from build123d import *

# Parameters (mm, degrees)
SKETCH1_R               = 15
SKETCH1_R_2             = 5
EXTRUDE_THIN1_DEPTH     = 50
SKETCH2_W               = 70
SKETCH2_H               = 30
BOSS_EXTRUDE1_DEPTH     = 16
SKETCH3_R               = 6
BOSS_EXTRUDE2_DEPTH     = 10
EXTRUDE_THIN2_DEPTH     = 12.5
FILLET1_R               = 30
BOSS_EXTRUDE3_DEPTH     = 10
CUT_EXTRUDE1_DEPTH      = 172.116081143
CUT_EXTRUDE1_DEPTH_BACK = 172.116081143
SKETCH6_R               = 10


with BuildPart() as part:
    # Sketch1 → Extrude-Thin1 (new, symmetric)
    with BuildSketch(Plane(origin=(0, 0, 0), x_dir=(0, 0, -1), z_dir=(1, 0, 0))):
        Circle(SKETCH1_R)
        Circle(SKETCH1_R_2, mode=Mode.SUBTRACT)
    extrude(amount=EXTRUDE_THIN1_DEPTH, both=True)

    # Sketch2 → Boss-Extrude1 (add)
    with BuildSketch(Plane(origin=(0, 0, 0), x_dir=(1, 0, 0), z_dir=(0, 1, 0))):
        Rectangle(SKETCH2_W, SKETCH2_H)
    extrude(amount=BOSS_EXTRUDE1_DEPTH)

    # Sketch3 → Boss-Extrude2 (add)
    with BuildSketch(Plane(origin=(0, 16, 0), x_dir=(1, 0, 0), z_dir=(0, 1, 0))):
        with Locations(Location((0, 0, 0), (0, 0, 270))):
            Circle(SKETCH3_R)
    extrude(amount=BOSS_EXTRUDE2_DEPTH)

    # Sketch4 → Extrude-Thin2 (add, symmetric)
    with BuildSketch(Plane(origin=(0, 0, 0), x_dir=(0, 0, -1), z_dir=(1, 0, 0))):
        Polygon((-14.175668382, 24.036944014), (10.301514998, 24.036944014), (42.733043078, 53.23603901), (154.74701088, 53.23603901), (154.74701088, 50.23603901), (43.884565313, 50.23603901), (11.453037232, 21.036944014), (-14.175668382, 21.036944014), align=None)
    extrude(amount=EXTRUDE_THIN2_DEPTH, both=True)

    # Fillet1
    # the kernel refuses this fillet: 30 mm, written as the material it adds along each edge
    with BuildSketch(Plane(origin=(12.5, 50.23603901, -43.884565313), x_dir=(0, -0.6691004351822665, 0.7431719906178524), z_dir=(-1, 0, 0))) as fillet1_piece_1:
        with BuildLine():
            CenterArc((FILLET1_R * 0.383840744794, -FILLET1_R), FILLET1_R, 90, 41.997673873)
            Line((-FILLET1_R * 0.285259690389, -FILLET1_R * 0.256828009382), (0, 0))
            Line((0, 0), (FILLET1_R * 0.383840744794, 0))
        make_face()
    extrude(amount=25)
    with BuildSketch(Plane(origin=(12.5, 24.036944014, -10.301514998), x_dir=(0, 0, 1), z_dir=(-1, 0, 0))) as fillet1_piece_2:
        with BuildLine():
            CenterArc((FILLET1_R * 0.383840744794, FILLET1_R), FILLET1_R, 228.002326127, 41.997673873)
            Line((-FILLET1_R * 0.285259690389, FILLET1_R * 0.256828009382), (0, 0))
            Line((0, 0), (FILLET1_R * 0.383840744794, 0))
        make_face()
    extrude(amount=25)
    # the kernel refuses this fillet: 30 mm, written as the material it takes off along each edge
    with BuildSketch(Plane(origin=(41.28805586, 53.23603901, -42.733043078), x_dir=(0, -0.6691004351822663, 0.7431719906178528), z_dir=(-1, 0, 0))) as fillet1_2_piece_1:
        with BuildLine():
            CenterArc((FILLET1_R * 0.383840744794, -FILLET1_R), FILLET1_R, 90, 41.997673873)
            Line((-FILLET1_R * 0.285259690389, -FILLET1_R * 0.256828009382), (0, 0))
            Line((0, 0), (FILLET1_R * 0.383840744794, 0))
        make_face()
    extrude(amount=82.576111719, mode=Mode.SUBTRACT)
    with BuildSketch(Plane(origin=(-41.28805586, 21.036944014, -11.453037232), x_dir=(0, 0, 1), z_dir=(1, 0, 0))) as fillet1_2_piece_2_section:
        with BuildLine():
            CenterArc((FILLET1_R * 0.383840744794, -FILLET1_R), FILLET1_R, 90, 41.997673873)
            Line((-FILLET1_R * 0.285259690389, -FILLET1_R * 0.256828009382), (0, 0))
            Line((0, 0), (FILLET1_R * 0.383840744794, 0))
        make_face()
    fillet1_2_piece_2 = extrude(amount=82.576111719, mode=Mode.PRIVATE)
    fillet1_2_piece_2 = fillet1_2_piece_2 - Plane(origin=(0, 22.678661346, 0), x_dir=(0, 0, 1), z_dir=(0, -1, 0)) * Cylinder(6, 212, mode=Mode.PRIVATE)
    add(fillet1_2_piece_2, mode=Mode.SUBTRACT)

    # Sketch5 → Boss-Extrude3 (add)
    with BuildSketch(Plane(origin=(50, 0, 0), x_dir=(0, 0, -1), z_dir=(1, 0, 0))):
        Polygon((-20.207259422, 0), (-10.103629711, -17.5), (10.103629711, -17.5), (20.207259422, 0), (10.103629711, 17.5), (-10.103629711, 17.5), align=None)
    boss_extrude3 = extrude(amount=-BOSS_EXTRUDE3_DEPTH)

    # Mirror1: Boss-Extrude3 across plane
    add(boss_extrude3.mirror(Plane(origin=(0, 0, 0), x_dir=(0, 0, 1), z_dir=(1, 0, 0))))

    # Sketch6 → Cut-Extrude1 (cut, two sides: drawn at the far end of the back side and taken through both)
    with BuildSketch(Plane(origin=(0, 0, 0), x_dir=(0, 0, -1), z_dir=(1, 0, 0)).offset(-CUT_EXTRUDE1_DEPTH_BACK)):
        Circle(SKETCH6_R)
    extrude(amount=CUT_EXTRUDE1_DEPTH + CUT_EXTRUDE1_DEPTH_BACK, mode=Mode.SUBTRACT)


solid = part.part
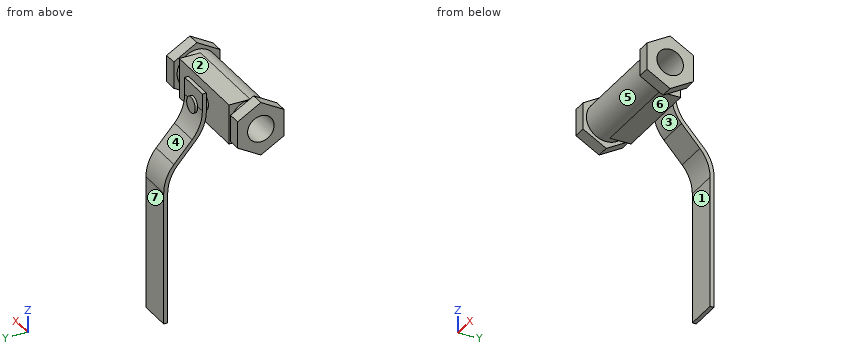
The listing builds one solid part. Answer for the finished solid, in the listing's coordinates (mm). Face numbers are marked on the shaded views. A direction names the side the tool comes from. Coordinates: 2 decimals unless noted, no trailing zeros. Order: outer loops, then holes, each group sorted by start corner. A loop starts at its lowest first (then second) coordinate and runs counter-clockwise, first axis right, second up.
Q1. Given P1, Ø8, axis at y = 8, z = 0, coming from the +X side; P2, Ø4, axis at x = 0.5, z = 7, coming from the +Y side; P3, Ø5, axis at x = 16.5, z = -90.5, coming from the +Y side; P4, Ø13, axis at x = -2.5, y = 5, coming from the +Z side, each flat-ended and moving along its own axis, determine where each tip first touches the part or whether it passes through.
Q2. Which of the six approach directions +Z, -Z, +X, -X, +Y, -Y give full straight-line access (tool end or side, diameter ignored) to the marked faces 5, 6 and 7?
Q3. Consider line 1 (Y direction, x = 9, z = 0); line 2 (Z direction, x = -24, y = 0); line 3 (Y direction, x = 22, z = 0). Determine where each line is inside the solid, lowest interval first.
Q4. For a pull along Y with two mould halves and no side action, classify the marked faces 1, 2, 3 and 4 as pulls with the +Y half, pulls with the -Y half, needs draft (parallel to the pull), parting line crosses it, or undercut.
Q5. A cutting plane is placed at D-D, the plane x = 0. Write down the section's boundary in (y, z), and give its area (3 significant figures).
Q6. A cutting plane is placed at A-A, the plane x = 27. Write down the section's boundary in (y, z), and give its area (3 significant figures).
Q7. A cutting plane is placed at C-C, the plane z = -137. Write down the section's boundary in (x, y).
Q8. A cutting plane is placed at B-B, the plane y = 6. Write down the section's boundary in (x, z), and give its area (3 significant figures).
Answers follow:
1. P1: stops at x = 50
1. P2: stops at y = 26
1. P3: passes through
1. P4: stops at z = 15
2. face 5: none
2. face 6: -Z, -Y
2. face 7: +Z, -Z, +X, -X, +Y
3. line 1: y = -15 to -10, 10 to 16, 21.04 to 24.06
3. line 2: z = -15 to -10, 10 to 15
3. line 3: y = -15 to -10, 10 to 16
4. face 1: pulls with the -Y half
4. face 2: needs draft
4. face 3: undercut
4. face 4: pulls with the +Y half
5. outline: (0, -15) - (16, -15) - (16, -6) - (21.66, -6) arc R30 ccw to (28.74, -20.01) - (42.53, -35.33) arc R30 cw to (50.24, -55.4) - (50.24, -154.75) - (53.24, -154.75) - (53.24, -54.25) arc R30 ccw to (45.53, -34.18) - (31.74, -18.86) arc R30 cw to (24.92, -6) - (26, -6) - (26, 6) - (24.04, 6) - (24.04, 14.18) - (21.04, 14.18) - (21.04, 6) - (16, 6) - (16, 15) - (0, 15) arc R15 ccw to start; hole circle Ø20 at (0, 0)
5. area: 1,140 mm2
6. outline: (0, -15) - (16, -15) - (16, 15) - (0, 15) arc R15 ccw to start; hole circle Ø20 at (0, 0)
6. area: 519 mm2
7. outline: (-12.5, 50.24) - (12.5, 50.24) - (12.5, 53.24) - (-12.5, 53.24) - close
8. outline: (-50, -16.74) - (-40, -16.74) - (-40, -13.75) - (-35, -13.75) - (-35, -15) - (35, -15) - (35, -13.75) - (40, -13.75) - (40, -16.74) - (50, -16.74) - (50, -8) - (-50, -8) - close; (-50, 8) - (50, 8) - (50, 16.74) - (40, 16.74) - (40, 13.75) - (35, 13.75) - (35, 15) - (-35, 15) - (-35, 13.75) - (-40, 13.75) - (-40, 16.74) - (-50, 16.74) - close
8. area: 1,440 mm2
